from build123d import *

# Parameters (mm, degrees)
F0_W = 26.6077592969
F0_H = 31.5558686852
F3_R = 5.08
F4_R = 5.08


with BuildPart() as f2:
    # F0 (on Top) → F2 (revolve)
    with BuildSketch(Plane.XY):
        with Locations((-13.3038796484, -15.7779343426)):
            Rectangle(F0_W, F0_H)
    revolve(axis=Axis((23.4335027635, -18.3920301497, 0), (0, -1, 0)))

    # F3
    f3_edges = [f2.edges().sort_by_distance(p)[0] for p in [
        (73.474765, 0, 0),
    ]]
    fillet(f3_edges, radius=F3_R)

    # F4
    f4_edges = [f2.edges().sort_by_distance(p)[0] for p in [
        (73.474765, -31.555869, 0),
    ]]
    fillet(f4_edges, radius=F4_R)


solid = f2.part
Work out the finished part from the listing and answer in its coordinate system (mm). Give positions to 0.01 mm unless a question says otherwise; leave off trailing zeros. Order: outer loops, then holes, each group sorted by start corner. A loop starts at its lowest first (then second) coordinate and runs counter-clockwise, first axis right, second up. Notation, with made-up numbers: (89.25, 47.5) -> (139.25, 47.5) arc R34 ccw to (139.25, 78.5) -> close; hole circle Ø11 at (54, -29). An arc over 180 degrees is marked (long way). Answer as a JSON object with one key per item and string values. Group by question number.
1. Consider line 1 along X through (y, z) = (-16, 0); line 2 along Z through (x, y) = (24, -26); line 3 along X through (y, z) = (-6.5, 9). Determine where each line is inside the solid, lowest interval first. Write a range as [from, to].
2. The mould has two halves that part along Z. Classify faces 1 (the flat face through (4, -31.556, 19)), 2 (the cylindrical face through (0.343, -15.628, 44.395)), 3 (the cylindrical face through (1.79, -15.56, 8.98)): released by +Z, released by -Z, zero draft, split by the parting line, or undercut.
3. Section B-B on y = -7 is taken. Determine the outline of the cut face in (x, z), plus the area to 3 significant figures.
4. Section C-C on y = -29 is taken. Determine the outline of the cut face in (x, z).
5. Flat-ended cylindrical pins translate along their axes: pin 1 Ø10 at (x, y) = (-3, -23.5) entering from +Z; pin 2 Ø1 at (y, z) = (-6, 23.5) entering from +X; pin 3 Ø12 at (y, z) = (-21, 9.5) entering from -X. Find the tip coordinate at first contact, or state that the pin passes through.
6. Section A-A on z = 0 is taken. Determine the outline of the cut face in (x, y), plus the area to 3 significant figures.
Result sheet:
{
 "1": {"line 1": "x = [-26.61, 0], [46.87, 73.47]", "line 2": "z = [-50.04, -23.43], [23.43, 50.04]", "line 3": "x = [-25.79, 1.8], [45.07, 72.66]"},
 "2": {"face 1": "zero draft", "face 2": "split by the parting line", "face 3": "undercut"},
 "3": {"outline": "circle Ø100.08 at (23.43, 0); hole circle Ø46.87 at (23.43, 0)", "area": "6,140 mm^2"},
 "4": {"outline": "circle Ø98.74 at (23.43, 0); hole circle Ø46.87 at (23.43, 0)"},
 "5": {"pin 1": "stops at z = 45.22", "pin 2": "stops at x = 67.88", "pin 3": "stops at x = -26.49"},
 "6": {"outline": "(-26.61, -26.48) arc R5.08 ccw to (-21.53, -31.56) -> (0, -31.56) -> (0, 0) -> (-21.53, 0) arc R5.08 ccw to (-26.61, -5.08) -> close; (46.87, -31.56) -> (68.39, -31.56) arc R5.08 ccw to (73.47, -26.48) -> (73.47, -5.08) arc R5.08 ccw to (68.39, 0) -> (46.87, 0) -> close", "area": "1,660 mm^2"}
}
